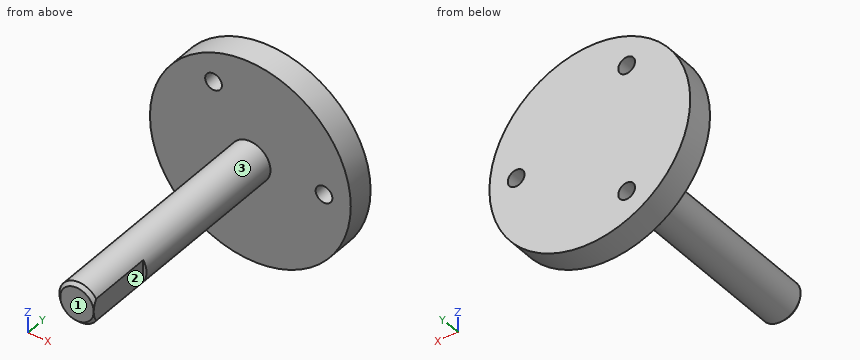
from build123d import *

# Parameters (mm, degrees)
CROQUIS1_W                                 = 3
CROQUIS1_H                                 = 39
CORTAR_EXTRUIR1_DEPTH                      = 10
CROQUIS4_R                                 = 15
SALIENTE_EXTRUIR1_DEPTH                    = 4
PERFORADOR_PARA_ROSCAR_PARA_MACHO_DE_ROS_D = 2.5
CHAFL_N1_SIZE                              = 0.5


with BuildPart() as part:
    # Croquis1 → Revolución1 (revolve)
    with BuildSketch(Plane.XY):
        with Locations((1.5, -19.5)):
            Rectangle(CROQUIS1_W, CROQUIS1_H)
    revolve(axis=Axis((0, -39, 0), (0, 1, 0)))

    # Croquis2 → Cortar-Extruir1 (cut)
    with BuildSketch(Plane.XZ.offset(39)):
        with BuildLine():
            Line((2.5, 1.658312395), (2.5, -1.658312395))
            ThreePointArc((2.5, -1.658312395), (3, 0), (2.5, 1.658312395))
        make_face()
    extrude(amount=-CORTAR_EXTRUIR1_DEPTH, mode=Mode.SUBTRACT)

    # Croquis4 → Saliente-Extruir1 (add)
    with BuildSketch(Plane(origin=(0, 0, 0), x_dir=(1, 0, 0), z_dir=(0, 1, 0))):
        with Locations(Location((0, 0, 0), (0, 0, 180))):
            Circle(CROQUIS4_R)
    extrude(amount=-SALIENTE_EXTRUIR1_DEPTH)

    # Perforador para roscar para macho de roscar para M3x0.51 (through all)
    with Locations(Plane(origin=(0, 0, 0), x_dir=(1, 0, 0), z_dir=(0, 1, 0))):
        with Locations((11, 0), (-5.5, -9.526279442), (-5.5, 9.526279442)):
            Hole(PERFORADOR_PARA_ROSCAR_PARA_MACHO_DE_ROS_D / 2)

    # Chaflán1
    chafl_n1_edges = [part.edges().sort_by_distance(p)[0] for p in [
        (-3, -39, 0),
    ]]
    chamfer(chafl_n1_edges, length=CHAFL_N1_SIZE - 0.0001)  # a hair under: the kernel refuses the full size


solid = part.part
Input: part model. Units: mm. Frame: model coordinates. Face numbers are marked on the shaded views. A direction names the side the tool comes from. Give positions to 0.01 mm unless a question says otherwise; leave off trailing zeros. Loops run counter-clockwise (first coordinate to the right, second up) from the corner with the lowest first, then second, coordinate; pieces in that order, holes last. Notation, with made-up numbers: (44, 57.5) -> (59, 57.5) arc R6 ccw to (59, 68.5) -> close; hole circle Ø5 at (75.5, 14.25). An arc over 180 degrees is marked (long way). Answer as a JSON object with one key per item and string values. Group by question number.
Item 1: Cut plane D-D, the plane x = 11. Return the cut outline in (y, z), and give its area (3 significant figures).
Item 2: Pin query (flat end, axial travel): P1, Ø2, axis at x = 11, z = 0, coming from the -Y side; P2, Ø3, axis at x = -5.5, z = 9.53, coming from the -Y side; P3, Ø2.5, axis at y = -32, z = -0.5, coming from the +X side; P4, Ø3, axis at x = -3.5, y = -28.5, coming from the -Z side. Return the tip coordinate at first contact, or that it passes through.
Item 3: Line query: probe 1 along Z at (x, y) = (-5.5, -2.8); probe 2 along Y at (x, z) = (9.5, -5.5); probe 3 along Z at (x, y) = (11, -2.1). Output: solid intervals per line, ascending.
Item 4: Reachability of the marked faces 1, 2 and 3 from +Z, -Z, +X, -X, +Y, -Y: full face, straight path, thin tool, end or side. Return the list, or none.
Item 5: Cut plane A-A, the plane x = 0. Return the cut outline in (y, z), and give its area (3 significant figures).
Item 6: Cut plane B-B, the plane x = -5.5. Return the cut outline in (y, z).
Item 7: Cut plane C-C, the plane z = -10.25. Return the cut outline in (x, y).
Checks:
{
 "1": {"outline": "(-4, -10.2) -> (0, -10.2) -> (0, -1.25) -> (-4, -1.25) -> close; (-4, 1.25) -> (0, 1.25) -> (0, 10.2) -> (-4, 10.2) -> close", "area": "71.6 mm²"},
 "2": {"P1": "passes through", "P2": "stops at y = -4", "P3": "stops at x = 2.5", "P4": "stops at z = -2.24"},
 "3": {"probe 1": "z = -13.96 to -10.78, -8.28 to 8.28, 10.78 to 13.96", "probe 2": "y = -4 to 0", "probe 3": "z = -10.2 to -1.25, 1.25 to 10.2"},
 "4": {"face 1": "+Z, -Z, +X, -X, -Y", "face 2": "+Z, -Z, +X, -Y", "face 3": "-Y"},
 "5": {"outline": "(-39, -2.5) -> (-38.5, -3) -> (-4, -3) -> (-4, -15) -> (0, -15) -> (0, 15) -> (-4, 15) -> (-4, 3) -> (-38.5, 3) -> (-39, 2.5) -> close", "area": "330 mm²"},
 "6": {"outline": "(-4, -13.96) -> (0, -13.96) -> (0, -10.78) -> (-4, -10.78) -> close; (-4, -8.28) -> (0, -8.28) -> (0, 8.28) -> (-4, 8.28) -> close; (-4, 10.78) -> (0, 10.78) -> (0, 13.96) -> (-4, 13.96) -> close"},
 "7": {"outline": "(-10.95, -4) -> (-6.52, -4) -> (-6.52, 0) -> (-10.95, 0) -> close; (-4.48, -4) -> (10.95, -4) -> (10.95, 0) -> (-4.48, 0) -> close"}
}
